Autodesk Inventor part; units mm, degrees
ref_plane "YZ Plane" through (0, 0, 0) normal (1, 0, 0) x (0, 1, 0)
ref_plane "XZ Plane" through (0, 0, 0) normal (0, 1, 0) x (-1, 0, 0)
ref_plane "XY Plane" through (0, 0, 0) normal (0, 0, 1) x (1, 0, 0)
sketch "Sketch1" plane through (0, 0, 0) normal (0, 0, 1) x (1, 0, 0)
  line L0 (0, 0) -> (0, 15.875)
  line L1 (0, 15.875) -> (0.7937, 15.875)
  line L2 (0.7937, 15.875) -> (0.7938, 0.7937)
  line L3 (0.7938, 0.7937) -> (15.875, 0.7937)
  line L4 (15.875, 0.7937) -> (15.875, 0)
  line L5 (15.875, 0) -> (0, 0)
  dimension "d0" = 15.875
  dimension "d1" = 0.7937
extrude "Extrusion1" add sketch "Sketch1" along normal blind 304.8
sketch "Sketch2" plane through (0.7938, 0.7937, 0) normal (0, 1, 0) x (1, 0, 0)
  line L0 (0, 0) -> (15.0812, 0)
  line L1 (15.0812, -304.8) -> (0, -304.8)
  line L2 (7.5406, 0) -> (7.5406, -304.8) construction
  circle A0 centre (7.5406, -9.525) radius 1.5875
  circle A1 centre (7.5406, -80.9625) radius 1.5875
  circle A2 centre (7.5406, -152.4) radius 1.5875
  circle A3 centre (7.5406, -223.8375) radius 1.5875
  circle A4 centre (7.5406, -295.275) radius 1.5875
  point P0 (-0.7938, 0)
  dimension "d4" = 9.525
  dimension "d5" = 3.175
  dimension "d6" = 304.8
  dimension "d9" = 71.4375
sketch "Sketch3" plane through (0.7938, 0.7937, 0) normal (1, 0, 0) x (0, 0, -1)
  line L0 (0, 15.0812) -> (0, 0)
  line L1 (-304.8, 0) -> (-304.8, 15.0812)
  line L2 (-304.8, 7.5406) -> (0, 7.5406) construction
  circle A0 centre (-9.525, 7.5406) radius 1.5875
  circle A1 centre (-80.9625, 7.5406) radius 1.5875
  circle A2 centre (-152.4, 7.5406) radius 1.5875
  circle A3 centre (-223.8375, 7.5406) radius 1.5875
  circle A4 centre (-295.275, 7.5406) radius 1.5875
  point P0 (0, -0.7937)
  dimension "d14" = 3.175
  dimension "d15" = 9.525
  dimension "d16" = 304.8
  dimension "d19" = 71.4375
extrude "Extrusion2" cut sketch "Sketch2" against normal through all
extrude "Extrusion3" cut sketch "Sketch3" against normal through all
properties part number "Hopper Bracing Right Bottom P9" material "Aluminum 6061"
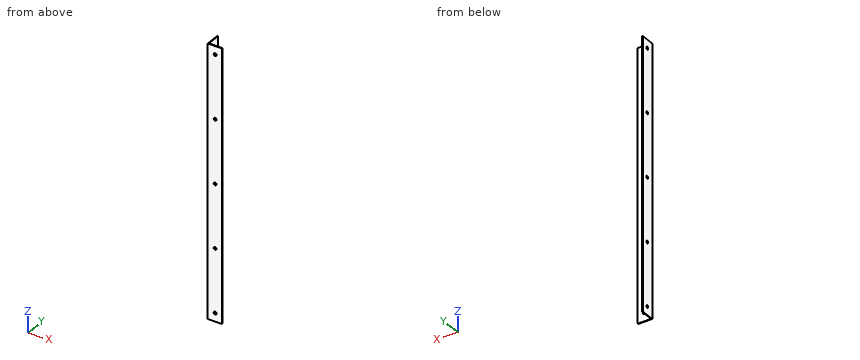
Build history of the part. All positions in model axes, mm. Round coordinates to 2 decimals unless told otherwise and drop trailing zeros. Loops run counter-clockwise (first coordinate to the right, second up) from the corner with the lowest first, then second, coordinate; pieces in that order, holes last.
Item 1: Pin check, flat tips, straight feed: P1, Ø1.5, axis at x = 11, z = 89.5, coming from the +Y side; P2, Ø1.9, axis at y = 8.33, z = 295.27, coming from the +X side; P3, Ø4.5, axis at y = 9.5, z = 150.5, coming from the +X side. Stop position of each tip, or through.
Item 2: Drill centre lines: line 1 along X through (y, z) = (0.3, 152.4) (3 decimals); line 2 along X through (y, z) = (13.75, 143). Where is each one in solid material? Low to high.
Item 3: Saw through at A-A (z = 128). List the corners of the cut face in (x, y) (3 decimals), then the cut area to 3 significant figures.
Item 4: Saw through at B-B (x = 12.5). List the corners of the cut face in (y, z).
Worked answers:
1. P1: stops at y = 0.79
1. P2: passes through
1. P3: stops at x = 0.79
2. line 1: x = 0 to 6.747, 9.922 to 15.875
2. line 2: x = 0 to 0.79
3. outline: (0, 0) - (15.875, 0) - (15.875, 0.794) - (0.794, 0.794) - (0.794, 15.875) - (0, 15.875) - close
3. area: 24.6 mm2
4. outline: (0, 0) - (0.79, 0) - (0.79, 304.8) - (0, 304.8) - close
